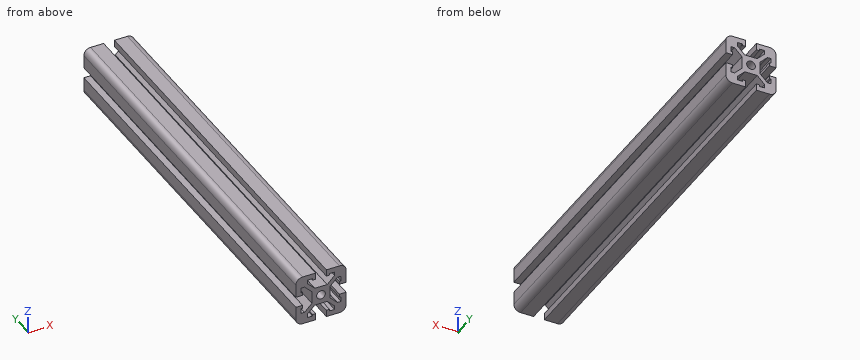
from build123d import *

# Parameters (mm, degrees)
F3_DEPTH = 304.8
F2_R     = 3.302
F4_DEPTH = 304.801
F5_R     = 5.08


with BuildPart() as f3:
    # F1 (on Front) → F3 (new body)
    with BuildSketch(Plane.XZ):
        Polygon((19.05, 19.05), (4.064, 19.05), (4.064, 13.97), (6.477, 13.97), (6.477, 15.24), (10.287, 15.24), (10.287, 13.97), (10.287, 12.442261), (4.702739, 6.858), (4.064, 6.858), (-4.064, 6.858), (-4.702739, 6.858), (-10.287, 12.442261), (-10.287, 13.97), (-10.287, 15.24), (-6.477, 15.24), (-6.477, 13.97), (-4.064, 13.97), (-4.064, 19.05), (-19.05, 19.05), (-19.05, 4.064), (-13.97, 4.064), (-13.97, 6.477), (-15.24, 6.477), (-15.24, 10.287), (-13.97, 10.287), (-12.442261, 10.287), (-6.858, 4.702739), (-6.858, 4.064), (-6.858, 0), (-6.858, -4.064), (-6.858, -4.702739), (-12.442261, -10.287), (-13.97, -10.287), (-15.24, -10.287), (-15.24, -6.477), (-13.97, -6.477), (-13.97, -4.064), (-19.05, -4.064), (-19.05, -19.05), (-4.064, -19.05), (-4.064, -13.97), (-6.477, -13.97), (-6.477, -15.24), (-10.287, -15.24), (-10.287, -13.97), (-10.287, -12.442261), (-4.702739, -6.858), (-4.064, -6.858), (0, -6.858), (4.064, -6.858), (4.702739, -6.858), (10.287, -12.442261), (10.287, -13.97), (10.287, -15.24), (6.477, -15.24), (6.477, -13.97), (4.064, -13.97), (4.064, -19.05), (19.05, -19.05), (19.05, -4.064), (13.97, -4.064), (13.97, -6.477), (15.24, -6.477), (15.24, -10.287), (13.97, -10.287), (12.442261, -10.287), (6.858, -4.702739), (6.858, -4.064), (6.858, 0), (6.858, 4.064), (6.858, 4.702739), (12.442261, 10.287), (13.97, 10.287), (15.24, 10.287), (15.24, 6.477), (13.97, 6.477), (13.97, 4.064), (19.05, 4.064), align=None)
    extrude(amount=F3_DEPTH)

    # F2 (on Front) → F4 (cut, through all)
    with BuildSketch(Plane.XZ):
        Circle(F2_R)
    extrude(amount=F4_DEPTH, mode=Mode.SUBTRACT)

    # F5
    f5_edges = [f3.edges().sort_by_distance(p)[0] for p in [
        (19.05, -152.4, 19.05),
        (-19.05, -152.4, 19.05),
        (19.05, -152.4, -19.05),
        (-19.05, -152.4, -19.05),
    ]]
    fillet(f5_edges, radius=F5_R)


solid = f3.part
Here's how the part is built. I have some questions about the finished solid (model axes, mm). Coordinates: 2 decimals unless noted, no trailing zeros. Order: outer loops, then holes, each group sorted by start corner. A loop starts at its lowest first (then second) coordinate and runs counter-clockwise, first axis right, second up. Notation, with made-up numbers: M -24,80 L -1,80 A22 cw -1,100 Z; hole C 4,38 d4. An arc over 180 degrees is marked long. Answer as CSV lines item,"result". Start each with the question number.
1. I want a section at A-A, the plane z = 0. Write out the boundary of the cut face in (x, y), and give its area (3 significant figures).
2. I need wall thicknesses on line 1 (Z direction, x = 4.5, y = -192.5); line 2 (X direction, y = -119, z = 0); line 3 (X direction, y = -207, z = 12.5). Which ranges of each line are inside material? Lowest first, please. Write a range as [from, to].
3. For pin 1 (3 mm diameter, centred on y = -211.5, z = 0, fed in from +X); pin 2 (0.6 mm diameter, centred on y = -89, z = -15, fed in from -X); pin 3 (4.5 mm diameter, centred on x = 1, y = -137, fed in from -Z); pin 4 (3 mm diameter, centred on x = -3, z = -11.5, fed in from -Y), each with a flat end and sliding along its axis, tell me the tip position at first contact or that it passes through.
4. I want a section at B-B, the plane x = 0. Write out the boundary of the cut face in (y, z).
Recorded:
1,outline,"M -6.86,-304.8 L -3.3,-304.8 L -3.3,0 L -6.86,0 Z; M 3.3,-304.8 L 6.86,-304.8 L 6.86,0 L 3.3,0 Z"
1,area,"2,170 mm2"
2,line 1,"z = [-19.05, -13.97], [-6.86, 6.86], [13.97, 19.05]"
2,line 2,"x = [-6.86, -3.3], [3.3, 6.86]"
2,line 3,"x = [-19.05, -10.29], [10.29, 19.05]"
3,pin 1,"stops at x = 6.86"
3,pin 2,"stops at x = -19"
3,pin 3,"stops at z = -6.86"
3,pin 4,"passes through"
4,outline,"M -304.8,-6.86 L 0,-6.86 L 0,-3.3 L -304.8,-3.3 Z; M -304.8,3.3 L 0,3.3 L 0,6.86 L -304.8,6.86 Z"
